CAD build for the part. Positions are in the model's coordinates, mm. A direction names the side the tool comes from. Round coordinates to 2 decimals unless told otherwise and drop trailing zeros. Write each loop counter-clockwise with the first axis right and the second up, starting at its lowest first coordinate (ties: lowest second). Pieces come first, ordered by that corner, then holes. Notation, with made-up numbers: (-0.75, 64.25) - (15.25, 64.25) arc R22 ccw to (15.25, 86.25) - close; hole circle Ø10 at (13, 47.5). An arc over 180 degrees is marked (long way). Put each result on its own line as item: value. Start each with the question number.
Item 1: Cut at D-D (y = 37). Give the cut face in (x, z), and give its area (3 significant figures).
Item 2: Cut at C-C (x = 1). Give the cut face in (y, z), and give its area (3 significant figures).
Item 3: Cut at A-A (y = 24). Give the cut face in (x, z).
Item 4: Pin check, flat tips, straight feed: pin 1 Ø11 at (y, z) = (20.5, 19) entering from +X; pin 2 Ø4 at (x, y) = (-7.5, 21) entering from -Z; pin 3 Ø1.5 at (x, y) = (-2.5, 35.5) entering from +Z. Stop position of each tip, or through.
Item 5: Drill centre lines: line 1 (Y direction, x = -10.75, z = -17.5); line 2 (X direction, y = 33, z = 0); line 3 (Z direction, x = -3, y = 9). Where is each one in solid material? Low to high. Write a range as from..to.
Item 6: Cut at B-B (z = 15.5). Give the cut face in (x, y).
Item 7: Mould opens along Z. For faces 4 (the flat face through (-6, 24, -12.5)), 5 (the flat face through (-6, 24, 12.5)), 6 (the cylindrical face through (-7.495, 23.664, -0.27)), 7 (the flat face through (-12.5, 24, 0)) say: released by +Z, released by -Z, zero draft, split by the parting line, or undercut.
Item 8: 3-axis set-ups, long thin cutter, end or side, ignore diameter. For faces 1 (the flat face through (-7.4, 0, -3)), 2 (the flat face through (-6.5, 24, -14)), 3 (the flat face through (-6.5, 24, 14)): which of +Z, -Z, +X, -X, +Y, -Y reach the whole face in a straight line?
```python
from build123d import *

# Parameters (mm, degrees)
SKETCH1_R           = 7.5
BOSS_EXTRUDE1_DEPTH = 48
BOSS_EXTRUDE2_DEPTH = 6
SKETCH3_R           = 2.6
CUT_EXTRUDE1_DEPTH  = 6
FILLET6_R           = 5
FILLET7_R           = 5
CUT_EXTRUDE4_DEPTH  = 55.465585465
FILLET9_R           = 2
FILLET11_R          = 2


with BuildPart() as part:
    # Sketch1 → Boss-Extrude1 (new body)
    with BuildSketch(Plane(origin=(0, 0, 0), x_dir=(1, 0, 0), z_dir=(0, 1, 0))):
        with BuildLine():
            Line((0, 12.5), (-12.5, 12.5))
            Line((-12.5, 12.5), (-12.5, -12.5))
            Line((-12.5, -12.5), (0, -12.5))
            ThreePointArc((0, -12.5), (12.5, 0), (0, 12.5))
        make_face()
        with Locations(Location((0, 0, 0), (0, 0, 270))):
            Circle(SKETCH1_R, mode=Mode.SUBTRACT)
    extrude(amount=BOSS_EXTRUDE1_DEPTH)

    # Sketch2 → Boss-Extrude2 (add)
    with BuildSketch(Plane.ZY.offset(12.5)):
        with BuildLine():
            Line((-17.5, 29), (-12.5, 29))
            Line((-12.5, 29), (-12.5, 19))
            Line((-12.5, 19), (-17.5, 19))
            ThreePointArc((-17.5, 19), (-22.5, 24), (-17.5, 29))
        make_face()
        with BuildLine():
            Line((17.5, 29), (12.5, 29))
            Line((12.5, 29), (12.5, 19))
            Line((12.5, 19), (17.5, 19))
            ThreePointArc((17.5, 19), (22.5, 24), (17.5, 29))
        make_face()
    extrude(amount=-BOSS_EXTRUDE2_DEPTH)

    # Sketch3 → Cut-Extrude1 (cut)
    with BuildSketch(Plane.ZY.offset(12.5)):
        with Locations((-17.5, 24)):
            Circle(SKETCH3_R)
        with Locations((17.5, 24)):
            Circle(SKETCH3_R)
    extrude(amount=-CUT_EXTRUDE1_DEPTH, mode=Mode.SUBTRACT)

    # Fillet6
    fillet6_edges = [part.edges().sort_by_distance(p)[0] for p in [
        (-9.5, 19, -12.5),
    ]]
    fillet(fillet6_edges, radius=FILLET6_R - 0.0001)  # a hair under: the kernel refuses the full size

    # Fillet7
    fillet7_edges = [part.edges().sort_by_distance(p)[0] for p in [
        (-9.5, 19, 12.5),
        (-9.5, 29, 12.5),
        (-9.5, 29, -12.5),
    ]]
    fillet(fillet7_edges, radius=FILLET7_R - 0.0001)  # a hair under: the kernel refuses the full size

    # Sketch5 → Cut-Extrude4 (cut, through all)
    with BuildSketch(Plane.XZ):
        Polygon((12.5, 12.5), (6.5, 12.5), (6.5, 4.06939799), (6.3, 4.06939799), (6.3, -4.06939799), (6.5, -4.06939799), (6.5, -12.5), (12.5, -12.5), align=None)
    extrude(amount=-CUT_EXTRUDE4_DEPTH, mode=Mode.SUBTRACT)

    # Fillet9
    fillet9_edges = [part.edges().sort_by_distance(p)[0] for p in [
        (6.5, 24, 10.677078252),
    ]]
    fillet(fillet9_edges, radius=FILLET9_R)

    # Fillet11
    fillet11_edges = [part.edges().sort_by_distance(p)[0] for p in [
        (6.5, 24, -10.677078252),
    ]]
    fillet(fillet11_edges, radius=FILLET11_R)


solid = part.part
```
Output values:
1. outline: (-12.5, -12.5) - (0, -12.5) arc R12.5 ccw to (5.36, -11.29) arc R2 ccw to (6.5, -9.49) - (6.5, -4.07) - (6.3, -4.07) arc R7.5 cw (long way) to (6.3, 4.07) - (6.5, 4.07) - (6.5, 9.49) arc R2 ccw to (5.36, 11.29) arc R12.5 ccw to (0, 12.5) - (-12.5, 12.5) - close
1. area: 295 mm2
2. outline: (0, -12.46) - (48, -12.46) - (48, -7.43) - (0, -7.43) - close; (0, 7.43) - (48, 7.43) - (48, 12.46) - (0, 12.46) - close
2. area: 483 mm2
3. outline: (-12.5, -22.5) - (-6.5, -22.5) - (-6.5, -20.1) - (-12.5, -20.1) - close; (-12.5, -14.9) - (-6.5, -14.9) - (-6.5, -12.5) - (0, -12.5) arc R12.5 ccw to (5.36, -11.29) arc R2 ccw to (6.5, -9.49) - (6.5, -4.07) - (6.3, -4.07) arc R7.5 cw (long way) to (6.3, 4.07) - (6.5, 4.07) - (6.5, 9.49) arc R2 ccw to (5.36, 11.29) arc R12.5 ccw to (0, 12.5) - (-6.5, 12.5) - (-6.5, 14.9) - (-12.5, 14.9) - close; (-12.5, 20.1) - (-6.5, 20.1) - (-6.5, 22.5) - (-12.5, 22.5) - close
4. pin 1: x = -6.5
4. pin 2: z = -22.4
4. pin 3: z = 12.5
5. line 1: 19..21.4, 26.6..29
5. line 2: -12.5..-7.5
5. line 3: -12.5..-6.87, 6.87..12.5
6. outline: (-12.5, 18.58) - (-6.5, 18.58) - (-6.5, 22.34) - (-12.5, 22.34) - close; (-12.5, 25.66) - (-6.5, 25.66) - (-6.5, 29.42) - (-12.5, 29.42) - close
7. face 4: released by -Z
7. face 5: released by +Z
7. face 6: undercut
7. face 7: zero draft
8. face 1: +Z, -Z, +X, -X, -Y
8. face 2: -Z, +X, +Y, -Y
8. face 3: +Z, +X, +Y, -Y
